```python
from build123d import *

# Parameters (mm, degrees)
EXTRUDE_1_DEPTH     = 109
EXTRUDE_2_DEPTH     = 18
SKETCH_3_W          = 25
SKETCH_3_H          = 11.25
CUT_EXTRUDE_1_DEPTH = 18
SKETCH_4_W          = 25
SKETCH_4_H          = 27
EXTRUDE_3_DEPTH     = 27
CUT_EXTRUDE_2_DEPTH = 122.166018853
CUT_EXTRUDE_3_DEPTH = 166.462013552
FILLET_1_R          = 3
CUT_EXTRUDE_4_DEPTH = 223.40244064


# Read off the part's stored shape, not the designer's step: Бобышка-Вытянуть2
with BuildPart() as part:
    # Эскиз1 → Бобышка-Вытянуть1 (new, symmetric)
    with BuildSketch(Plane(origin=(0, 0, 0), x_dir=(0, 0, -1), z_dir=(1, 0, 0))):
        with BuildLine():
            Line((11, 0), (25.25, 0))
            Line((25.25, 0), (25.25, -9))
            Line((25.25, -9), (-25.25, -9))
            Line((-25.25, -9), (-25.25, 0))
            Line((-25.25, 0), (-11, 0))
            ThreePointArc((-11, 0), (0, 6), (11, 0))
        make_face()
    extrude(amount=EXTRUDE_1_DEPTH, both=True)

    # Бобышка-Вытянуть2 outline → Бобышка-Вытянуть2 (add)
    with BuildSketch(Plane(origin=(0, 0, 0), x_dir=(1, 0, 0), z_dir=(0, 1, 0))):
        Polygon((16, 11), (20.656976684, -11), (29.856406461, -11), (25.199429777, 11), align=None)
        Polygon((-29.856406461, -11), (-20.656976684, -11), (-16, 11), (-25.199429777, 11), align=None)
        Polygon((78.012123179, -10.999996132), (86.400679256, -10.994643711), (93.506557878, -2.272856192), (100.623560797, -10.985568626), (109.012116871, -10.980216204), (93.499996845, 8.009889964), align=None)
        Polygon((64.623554487, -11.008538874), (73.012110561, -11.003186452), (57.499990534, 7.986919716), (42.012116871, -11.02296638), (50.400672946, -11.017613959), (57.506551567, -2.29582644), align=None)
        Polygon((-109.012116871, -10.980216204), (-100.623560797, -10.985568626), (-93.506557878, -2.272856192), (-86.400679256, -10.994643711), (-78.012123179, -10.999996132), (-93.499996845, 8.009889964), align=None)
        Polygon((-73.012110561, -11.003186452), (-64.623554487, -11.008538874), (-57.506551567, -2.29582644), (-50.400672946, -11.017613959), (-42.012116871, -11.02296638), (-57.499990534, 7.986919716), align=None)
    extrude(amount=EXTRUDE_2_DEPTH)

    # Эскиз3 → Вырез-Вытянуть1 (cut)
    with BuildSketch(Plane(origin=(0, 0, 0), x_dir=(1, 0, 0), z_dir=(0, 1, 0))):
        with Locations((0, 19.625)):
            Rectangle(SKETCH_3_W, SKETCH_3_H)
        with Locations((0, -19.625)):
            Rectangle(SKETCH_3_W, SKETCH_3_H)
    extrude(amount=-CUT_EXTRUDE_1_DEPTH, mode=Mode.SUBTRACT)

    # Эскиз4 → Бобышка-Вытянуть3 (add)
    with BuildSketch(Plane.XZ.offset(9)):
        with Locations((38, 0)):
            Rectangle(SKETCH_4_W, SKETCH_4_H)
        with Locations((-38, 0)):
            Rectangle(SKETCH_4_W, SKETCH_4_H)
    extrude(amount=EXTRUDE_3_DEPTH)

    # Эскиз6 → Вырез-Вытянуть2 (cut, through all)
    with BuildSketch(Plane.XY.offset(13.5)):
        Polygon((-50.5, -9), (-50.5, -36), (-44.5, -36), align=None)
        Polygon((-25.5, -36), (-31.5, -36), (-25.5, -9), align=None)
        Polygon((25.5, -9), (25.5, -36), (31.5, -36), align=None)
        Polygon((50.5, -36), (44.5, -36), (50.5, -9), align=None)
    extrude(amount=-CUT_EXTRUDE_2_DEPTH, mode=Mode.SUBTRACT)

    # Эскиз5 → Вырез-Вытянуть3 (cut, through all)
    with BuildSketch(Plane.ZY.offset(50.5)):
        Polygon((-13.5, -9), (-13.5, -36), (-6.5, -36), align=None)
        Polygon((13.5, -36), (6.5, -36), (13.5, -9), align=None)
    extrude(amount=-CUT_EXTRUDE_3_DEPTH, mode=Mode.SUBTRACT)

    # Скругление1
    fillet_1_edges = [part.edges().sort_by_distance(p)[0] for p in [
        (-38, -36, -6.5),
        (38, -36, -6.5),
        (-38, -36, 6.5),
        (38, -36, 6.5),
    ]]
    fillet(fillet_1_edges, radius=FILLET_1_R)

    # Эскиз8 → Вырез-Вытянуть4 (cut, through all)
    with BuildSketch(Plane(origin=(109, 0, 0), x_dir=(0, 0, -1), z_dir=(1, 0, 0))):
        with BuildLine():
            Line((-22.75, -9), (-25.25, -9))
            Line((-25.25, -9), (-25.25, 0))
            Line((-25.25, 0), (-22.75, 0))
            ThreePointArc((-22.75, 0), (-18.25, -4.5), (-22.75, -9))
        make_face()
        with BuildLine():
            Line((22.75, -9), (25.25, -9))
            Line((25.25, -9), (25.25, 0))
            Line((25.25, 0), (22.75, 0))
            ThreePointArc((22.75, 0), (18.25, -4.5), (22.75, -9))
        make_face()
    extrude(amount=-CUT_EXTRUDE_4_DEPTH, mode=Mode.SUBTRACT)


solid = part.part
```
For this review, take the finished solid that the model builds, in its own axes (mm). A direction names the side the tool comes from. Round coordinates to 2 decimals unless told otherwise and drop trailing zeros. Write each loop counter-clockwise with the first axis right and the second up, starting at its lowest first coordinate (ties: lowest second). Pieces come first, ordered by that corner, then holes. Notation, with made-up numbers: (-2, 44) -> (45, 44) arc R31 ccw to (45, 73) -> close; hole circle Ø11 at (45, 41.5). An arc over 180 degrees is marked (long way). One line per question, with ' | ' between items. Start each with the question number.
1) Wall thickness on line 1 along Z through (x, y) = (-10, -6); line 2 along Y through (x, z) = (-88.5, -13.5); line 3 along Z through (x, y) = (70, -4): over which ranges is each line inside the solid? List them lowest first.
2) Mouldability with a two-part tool opening along X and no side actions: class faces 1 (the flat face through (-109, -3, 0)), 2 (the flat face through (48.125, -19.689, 0.189)), 3 (the flat face through (38, -36, 0)), 4 (the flat face through (18.296, 10.874, -0.154)) as +X half, -X half, draft (parallel to the pull), parting line (faces both ways), or undercut.
3) Machinability: for faces 5 (the flat face through (-12.5, -4, -16)), 6 (the flat face through (2, 0, -13)), 7 (the flat face through (37.825, -21.55, -10.246)), which of the approach directions +Z, -Z, +X, -X, +Y, -Y give a long, thin tool a straight path to every point of the face, cutting with its end or side? Answer none if there is none.
4) For pin 1 Ø4.5 at (y, z) = (-5, 17.5) entering from +X; pin 2 Ø9.5 at (x, z) = (26, -14.5) entering from +Y; pin 3 Ø4 at (x, y) = (-84.5, -2.5) entering from +Z; pin 4 Ø10 at (x, z) = (-7, -16.5) entering from -Y, all flat-tipped, find the tip position at first contact; note any pin that passes through.
5) Add section B-B (y = -18.5). Write out the cut boundary in (x, z).
6) Add section A-A (y = -4.5). Write out the cut boundary in (x, z), and give its area (3 significant figures).
Reported:
1) line 1: z = -14 to 14 | line 2: y = -9 to 0 | line 3: z = -18.28 to 18.28
2) face 1: -X half | face 2: +X half | face 3: draft | face 4: undercut
3) face 5: -Z, +Y, -Y | face 6: -Z, +X, -X, +Y | face 7: -Z, +X, -X, -Y
4) pin 1: stops at x = 109 | pin 2: stops at y = 18 | pin 3: stops at z = 20.69 | pin 4: stops at y = -9
5) outline: (-48.39, -11.04) -> (-27.61, -11.04) -> (-27.61, 11.04) -> (-48.39, 11.04) -> close; (27.61, -11.04) -> (48.39, -11.04) -> (48.39, 11.04) -> (27.61, 11.04) -> close
6) outline: (-109, -18.25) -> (-12.5, -18.25) -> (-12.5, -14) -> (12.5, -14) -> (12.5, -18.25) -> (109, -18.25) -> (109, 18.25) -> (12.5, 18.25) -> (12.5, 14) -> (-12.5, 14) -> (-12.5, 18.25) -> (-109, 18.25) -> close | area: 7,740 mm²
